Model file for the job. Use its own axes, mm. Face numbers are marked on the shaded views. A direction names the side the tool comes from. Coordinates: 2 decimals unless noted, no trailing zeros. Loops run counter-clockwise (first coordinate to the right, second up) from the corner with the lowest first, then second, coordinate; pieces in that order, holes last. Notation, with made-up numbers: (50.5, 43) - (91.5, 43) arc R24 cw to (91.5, 56) - close; hole circle Ø4 at (73, 50). An arc over 180 degrees is marked (long way). Write each question's results on one line, items separated by ' | '. Start each with the question number.
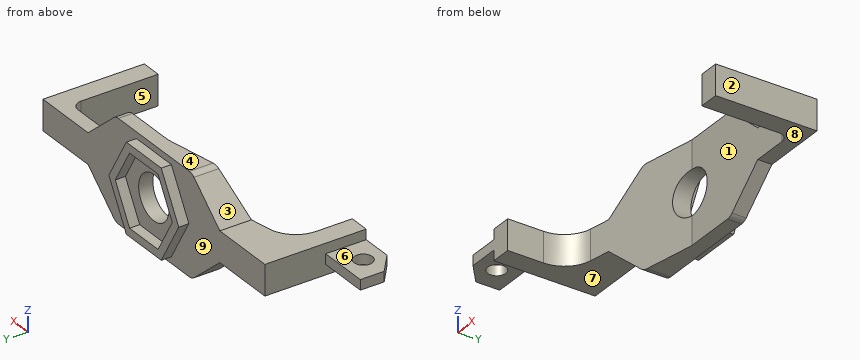
```python
from build123d import *

# Parameters (mm, degrees)
BOSS_EXTRUDE1_DEPTH      = 100
FILLET1_R                = 30
FILLET2_R                = 10
CUT_EXTRUDE1_DEPTH       = 100
CUT_EXTRUDE2_DEPTH       = 100
CUT_EXTRUDE3_DEPTH       = 100
CUT_EXTRUDE4_DEPTH       = 100
FILLET3_R                = 10
SKETCH9_R                = 22
CUT_EXTRUDE5_DEPTH       = 100
BOSS_EXTRUDE2_DEPTH      = 10
SKETCH11_R               = 22
CUT_EXTRUDE6_DEPTH       = 10
CUT_EXTRUDE7_DEPTH       = 10
BOSS_EXTRUDE3_DEPTH      = 5
BOSS_EXTRUDE3_DEPTH_BACK = 5
CUT_EXTRUDE10_DEPTH      = 240.057846604
CUT_EXTRUDE10_DEPTH_BACK = 240.057846604
SKETCH15_R               = 9


with BuildPart() as part:
    # Sketch2 → Boss-Extrude1 (new body)
    with BuildSketch(Plane.XY):
        Polygon((160, 0), (-160, 0), (-160, -100), (-140, -100), (-140, -39.427371229), (0, -14), (140, -14), (140, -100), (160, -100), align=None)
    extrude(amount=BOSS_EXTRUDE1_DEPTH)

    # Fillet1
    fillet1_edges = [part.edges().sort_by_distance(p)[0] for p in [
        (-140, -39.427371229, 50),
    ]]
    fillet(fillet1_edges, radius=FILLET1_R)

    # Fillet2
    fillet2_edges = [part.edges().sort_by_distance(p)[0] for p in [
        (140, -14, 50),
    ]]
    fillet(fillet2_edges, radius=FILLET2_R)

    # Sketch5 → Cut-Extrude1 (cut)
    with BuildSketch(Plane(origin=(0, 0, 0), x_dir=(1, 0, 0), z_dir=(0, 1, 0))):
        Polygon((-160, 0), (-160, -35), (-95, -35), (-55, 0), align=None)
    extrude(amount=-CUT_EXTRUDE1_DEPTH, mode=Mode.SUBTRACT)

    # Sketch6 → Cut-Extrude2 (cut)
    with BuildSketch(Plane(origin=(0, 0, 0), x_dir=(1, 0, 0), z_dir=(0, 1, 0))):
        Polygon((-160, -100), (-160, -65), (-95, -65), (-55, -100), align=None)
    extrude(amount=-CUT_EXTRUDE2_DEPTH, mode=Mode.SUBTRACT)

    # Sketch7 → Cut-Extrude3 (cut)
    with BuildSketch(Plane(origin=(0, 0, 0), x_dir=(1, 0, 0), z_dir=(0, 1, 0))):
        Polygon((160, 0), (160, -34.999520122), (95, -34.999520122), (55, 0), align=None)
    extrude(amount=-CUT_EXTRUDE3_DEPTH, mode=Mode.SUBTRACT)

    # Sketch8 → Cut-Extrude4 (cut)
    with BuildSketch(Plane(origin=(0, 0, 0), x_dir=(1, 0, 0), z_dir=(0, 1, 0))):
        Polygon((160, -100), (160, -65), (95, -65), (55, -100), align=None)
    extrude(amount=-CUT_EXTRUDE4_DEPTH, mode=Mode.SUBTRACT)

    # Fillet3
    fillet3_edges = [part.edges().sort_by_distance(p)[0] for p in [
        (55, -7, 100),
        (-55, -11.994662206, 0),
        (-55, -11.994662206, 100),
        (55, -7, 0),
    ]]
    fillet(fillet3_edges, radius=FILLET3_R)

    # Sketch9 → Cut-Extrude5 (cut)
    with BuildSketch(Plane(origin=(0, 0, 0), x_dir=(1, 0, 0), z_dir=(0, 1, 0))):
        with Locations(Location((0, -50, 0), (0, 0, 180))):
            Circle(SKETCH9_R)
    extrude(amount=-CUT_EXTRUDE5_DEPTH, mode=Mode.SUBTRACT)

    # Sketch10 → Boss-Extrude2 (add)
    with BuildSketch(Plane(origin=(0, 0, 0), x_dir=(1, 0, 0), z_dir=(0, 1, 0))):
        Polygon((-25.182222271, -6.383111579), (-50.364444542, -50), (-25.182222271, -93.616888421), (25.182222271, -93.616888421), (50.364444542, -50), (25.182222271, -6.383111579), align=None)
    extrude(amount=BOSS_EXTRUDE2_DEPTH)

    # Sketch11 → Cut-Extrude6 (cut)
    with BuildSketch(Plane(origin=(0, 10, 0), x_dir=(1, 0, 0), z_dir=(0, 1, 0))):
        with Locations(Location((0, -50, 0), (0, 0, 180))):
            Circle(SKETCH11_R)
    extrude(amount=-CUT_EXTRUDE6_DEPTH, mode=Mode.SUBTRACT)

    # Sketch12 → Cut-Extrude7 (cut)
    with BuildSketch(Plane(origin=(0, 10, 0), x_dir=(1, 0, 0), z_dir=(0, 1, 0))):
        Polygon((41.126840235, -50), (20.563420118, -14.383111579), (-20.563420118, -14.383111579), (-41.126840235, -50), (-20.563420118, -85.616888421), (20.563420118, -85.616888421), align=None)
    extrude(amount=-CUT_EXTRUDE7_DEPTH, mode=Mode.SUBTRACT)

    # Sketch14 → Boss-Extrude3 (add, two sides: drawn at the far end of the back side and taken through both)
    with BuildSketch(Plane.XY.offset(50).offset(-BOSS_EXTRUDE3_DEPTH_BACK)):
        Polygon((-160, -100), (-160, -60), (-210, -60), (-210.056311552, -83.454778124), (-190, -100), align=None)
    extrude(amount=BOSS_EXTRUDE3_DEPTH + BOSS_EXTRUDE3_DEPTH_BACK)

    # Sketch15 → Cut-Extrude10 (cut, two sides: drawn at the far end of the back side and taken through both)
    with BuildSketch(Plane.XY.offset(55).offset(-CUT_EXTRUDE10_DEPTH_BACK)):
        with Locations(Location((-185, -80, 0), (0, 0, 180))):
            Circle(SKETCH15_R)
    extrude(amount=CUT_EXTRUDE10_DEPTH + CUT_EXTRUDE10_DEPTH_BACK, mode=Mode.SUBTRACT)


solid = part.part
```
Q1. Pin check, flat tips, straight feed: pin 1 (11 mm diameter, centred on x = -190.5, z = 52.5, fed in from +Y); pin 2 (6 mm diameter, centred on y = -4, z = 29.5, fed in from -X); pin 3 (10 mm diameter, centred on y = -82.5, z = 53, fed in from -X); pin 4 (5 mm diameter, centred on x = 0, y = 7, fed in from -Z). Stop position of each tip, or through.
Q2. Cut at C-C (x = -37). List the corners of the cut face in (y, z).
Q3. Cut at D-D (x = 115). List the corners of the cut face in (y, z), and give its area (3 significant figures).
Q4. Drill centre lines: L1, parallel to Z at x = -9.5, y = 4.5; L2, parallel to Y at x = -185, z = 52; L3, parallel to X at y = -8, z = 50. Where is each one in solid material? Low to high. Write a range as from..to.
Q5. Which spindle directions (+Z, -Z, +X, -X, +Y, -Y) get a long thin tool onto all of the face, cutting with end or side? Do the marked faces 5, 6, 7, 8 and 9. Say none if no direction does.
Q6. Cut at A-A (x = -185). List the corners of the cut face in (y, z), and give its area (3 significant figures).
Q7. Mould opens along X. For the marked faces 1, 2, 3 and 4 say: +X half, -X half, draft (parallel to the pull), parting line (faces both ways), or undercut.
Q8. Cut at B-B (y = -80). List the corners of the cut face in (x, z).
Check result:
1) pin 1: y = -60 | pin 2: x = -92.14 | pin 3: x = -210.06 | pin 4: z = 6.38
2) outline: (-20.72, 0) - (0, 0) - (0, 26.85) - (10, 26.85) - (10, 42.85) - (0, 42.85) - (0, 57.15) - (10, 57.15) - (10, 73.15) - (0, 73.15) - (0, 100) - (-20.72, 100) - close
3) outline: (-14, 35) - (0, 35) - (0, 65) - (-14, 65) - close | area: 420 mm²
4) L1: 6.38..14.38, 85.62..93.62 | L2: -100..-89, -71..-60 | L3: -160..-22, 22..160
5) face 5: +Z, -Z, -Y | face 6: +Z, -X, +Y, -Y | face 7: -Z, -X, +Y, -Y | face 8: -Z, +X, +Y, -Y | face 9: +Y
6) outline: (-100, 45) - (-89, 45) - (-89, 55) - (-100, 55) - close; (-71, 45) - (-60, 45) - (-60, 55) - (-71, 55) - close | area: 220 mm²
7) face 1: undercut | face 2: +X half | face 3: -X half | face 4: draft
8) outline: (-210.05, 45) - (-194, 45) - (-194, 55) - (-210.05, 55) - close; (-176, 45) - (-160, 45) - (-160, 35) - (-140, 35) - (-140, 65) - (-160, 65) - (-160, 55) - (-176, 55) - close; (140, 35) - (160, 35) - (160, 65) - (140, 65) - close
